Work out the finished part from the listing and answer in its coordinate system (mm). Face numbers are marked on the shaded views. A direction names the side the tool comes from. Round coordinates to 2 decimals unless told otherwise and drop trailing zeros. Order: outer loops, then holes, each group sorted by start corner. A loop starts at its lowest first (then second) coordinate and runs counter-clockwise, first axis right, second up. Notation, with made-up numbers: M -23.75,53.5 L 5.25,53.5 A17 cw 5.25,75.5 Z; hole C 55.25,-10.75 d10. An arc over 180 degrees is marked long. Return JSON: item names as keys, results as strings.
from build123d import *

# Parameters (mm, degrees)
ESQUISSE2_W                                    = 72
ESQUISSE2_H                                    = 14
BOSS_EXTRU_1_DEPTH                             = 41
ESQUISSE12_W                                   = 9
ESQUISSE12_H                                   = 20
BOSS_EXTRU_6_DEPTH                             = 14
FRAISAGE_POUR_VIS_T_TE_FRAIS_E_M41_D           = 4.3
FRAISAGE_POUR_VIS_T_TE_FRAIS_E_M41_CSINK_D     = 9.4
FRAISAGE_POUR_VIS_T_TE_FRAIS_E_M41_CSINK_ANGLE = 90
ENL_V_MAT_EXTRU_3_REACH                        = 95.798
ESQUISSE6_W                                    = 20
ESQUISSE6_H                                    = 10
ESQUISSE5_W                                    = 5.5
ESQUISSE5_H                                    = 50
ENL_V_MAT_EXTRU_2_DEPTH                        = 7
CHANFREIN1_SIZE                                = 2
ESQUISSE16_W                                   = 20
ESQUISSE16_H                                   = 7
BOSS_EXTRU_7_DEPTH                             = 10
ENL_V_START                                    = -14
ENL_V_MAT_EXTRU_4_DEPTH                        = 14
ENL_V_MAT_EXTRU_5_DEPTH                        = 7.5
CHANFREIN2_SIZE                                = 2
CONG_3_R                                       = 3


with BuildPart() as part:
    # Esquisse2 → Boss.-Extru.1 (new, symmetric)
    with BuildSketch(Plane.XY):
        Rectangle(ESQUISSE2_W, ESQUISSE2_H)
    extrude(amount=BOSS_EXTRU_1_DEPTH, both=True)

    # Esquisse12 → Boss.-Extru.6 (add)
    with BuildSketch(Plane(origin=(0, 7, 0), x_dir=(1, 0, 0), z_dir=(0, 1, 0))):
        with Locations((40.5, 0)):
            Rectangle(ESQUISSE12_W, ESQUISSE12_H)
    extrude(amount=-BOSS_EXTRU_6_DEPTH)

    # Fraisage pour vis à tête fraisée M41 (through all)
    with Locations(Plane(origin=(0, 7, 0), x_dir=(1, 0, 0), z_dir=(0, 1, 0))):
        with Locations((32.5, 0), (7.5, 0)):
            CounterSinkHole(FRAISAGE_POUR_VIS_T_TE_FRAIS_E_M41_D / 2, FRAISAGE_POUR_VIS_T_TE_FRAIS_E_M41_CSINK_D / 2, counter_sink_angle=FRAISAGE_POUR_VIS_T_TE_FRAIS_E_M41_CSINK_ANGLE)

    # Esquisse6 → Enlèv. mat.-Extru.3 (cut, up to next)
    with BuildSketch(Plane.XY.offset(41), mode=Mode.PRIVATE) as enl_v_mat_extru_3_sk1:
        with Locations((-18, -2)):
            Rectangle(ESQUISSE6_W, ESQUISSE6_H)
    enl_v_mat_extru_3_tool1 = extrude(enl_v_mat_extru_3_sk1.sketch, amount=-ENL_V_MAT_EXTRU_3_REACH, mode=Mode.PRIVATE) & part.part
    add(enl_v_mat_extru_3_tool1.solids().sort_by_distance((-18, -2, 41))[0], mode=Mode.SUBTRACT)

    # Esquisse5 → Enlèv. mat.-Extru.2 (cut)
    with BuildSketch(Plane(origin=(0, -7, 0), x_dir=(1, 0, 0), z_dir=(0, 1, 0))):
        with Locations((-33.25, 0)):
            Rectangle(ESQUISSE5_W, ESQUISSE5_H)
    extrude(amount=ENL_V_MAT_EXTRU_2_DEPTH, mode=Mode.SUBTRACT)

    # Chanfrein1
    chanfrein1_edges = [part.edges().sort_by_distance(p)[0] for p in [
        (0, 7, -41),
        (0, 7, 41),
    ]]
    chamfer(chanfrein1_edges, length=CHANFREIN1_SIZE)

    # Esquisse16 → Boss.-Extru.7 (add)
    with BuildSketch(Plane.XZ.offset(-3)):
        with Locations((-18, -37.5)):
            Rectangle(ESQUISSE16_W, ESQUISSE16_H)
    boss_extru_7 = extrude(amount=BOSS_EXTRU_7_DEPTH)

    # Symétrie1: Boss.-Extru.7 across plane
    add(boss_extru_7.mirror(Plane.XY))

    # Esquisse17 → Enlèv. mat.-Extru.4 (cut)
    with BuildSketch(Plane(origin=(0, 7, 0), x_dir=(1, 0, 0), z_dir=(0, 1, 0)).offset(ENL_V_START)):
        Polygon((13.342024655, -41), (21.739180223, -33.8), (7.912562911, -33.8), (-0.484592656, -41), align=None)
    extrude(amount=ENL_V_MAT_EXTRU_4_DEPTH, mode=Mode.SUBTRACT)

    # Esquisse18 → Enlèv. mat.-Extru.5 (cut)
    with BuildSketch(Plane(origin=(0, 7, 0), x_dir=(1, 0, 0), z_dir=(0, 1, 0))):
        Polygon((7.912562911, -33.8), (36, -10), (36, -21.716038419), (21.739180223, -33.8), align=None)
    extrude(amount=-ENL_V_MAT_EXTRU_5_DEPTH, mode=Mode.SUBTRACT)

    # Chanfrein2
    chanfrein2_edges = [part.edges().sort_by_distance(p)[0] for p in [
        (14.825871567, -0.5, 33.8),
        (36, -0.5, 15.858019209),
    ]]
    chamfer(chanfrein2_edges, length=CHANFREIN2_SIZE)

    # Congé3
    cong_3_edges = [part.edges().sort_by_distance(p)[0] for p in [
        (45, 0, 10),
        (45, 0, -10),
    ]]
    fillet(cong_3_edges, radius=CONG_3_R)


solid = part.part
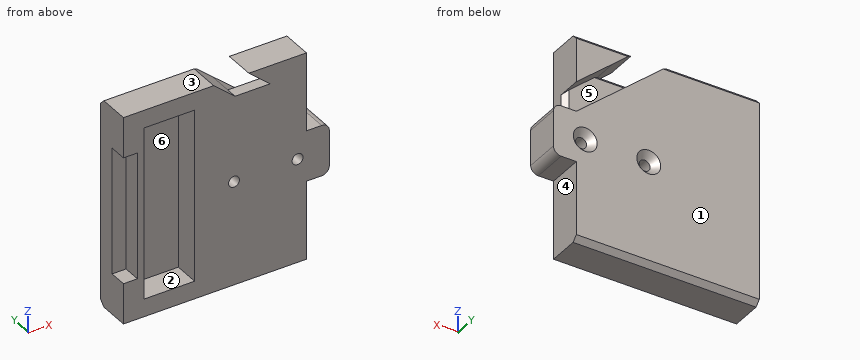
Item 1: Each of these flat-tipped pins is pushed along its axis until it touches: pin 1 (6 mm diameter, centred on x = 4, y = 1.5, fed in from +Z); pin 2 (5 mm diameter, centred on x = 39.5, y = -2, fed in from -Z); pin 3 (1.8 mm diameter, centred on x = 40, y = -0.5, fed in from +Z). Where does it stop, or does it pass through?
Output:
{"pin 1": "stops at z = 39.73", "pin 2": "stops at z = -10", "pin 3": "stops at z = 10"}
Item 2: Find section D-D (x = 32.5). Determine the outline of the cut face in (y, z), plus the area to 3 significant figures.
Output:
{"outline": "M -7,-41 L 5,-41 L 7,-39 L 7,-4.7 L 4.45,-2.15 L -7,-2.15 Z; M -7,2.15 L 4.45,2.15 L 7,4.7 L 7,12.97 L -0.5,12.97 L -0.5,24.68 L 7,24.68 L 7,39 L 5,41 L -7,41 Z", "area": "989 mm^2"}
Item 3: The mould has two halves that part along Z. Classify the marked faces 1, 2 and 3: pulls with the +Z half, pulls with the -Z half, needs draft (parallel to the pull), parting line crosses it, or undercut.
Output:
{"face 1": "needs draft", "face 2": "undercut", "face 3": "pulls with the +Z half"}
Item 4: Which of the six approach directions +Z, -Z, +X, -X, +Y, -Y give full straight-line access (tool end or side, diameter ignored) to the marked faces 4, 5 and 6?
Output:
{"face 4": "-Z, +X, +Y, -Y", "face 5": "+Y", "face 6": "-Y"}
Item 5: Find section A-A (y = 1.5). Determine the outline of the cut face in (x, z).
Output:
{"outline": "M -36,-41 L 36,-41 L 36,-10 L 42,-10 A3 ccw 45,-7 L 45,7 A3 ccw 42,10 L 36,10 L 7.91,33.8 L -0.48,41 L -36,41 Z; M 13.34,41 L 21.74,33.8 L 36,21.72 L 36,41 Z; hole M -28,-34 L -8,-34 L -8,34 L -28,34 Z; hole C 7.5,0 d4.3; hole C 32.5,0 d4.3"}
Item 6: Find section B-B (z = 0). Determine the outline of the cut face in (x, y).
Output:
{"outline": "M -36,0 L -30.5,0 L -30.5,-7 L -28,-7 L -28,3 L -8,3 L -8,-7 L 5.35,-7 L 5.35,4.45 L 2.8,7 L -36,7 Z; M 9.65,-7 L 30.35,-7 L 30.35,4.45 L 27.8,7 L 12.2,7 L 9.65,4.45 Z; M 34.65,-7 L 45,-7 L 45,7 L 37.2,7 L 34.65,4.45 Z"}
Item 7: Find section C-C (z = -19.5). Determine the outline of the cut face in (x, y), plus the area to 4 significant figures.
Output:
{"outline": "M -36,0 L -30.5,0 L -30.5,-7 L -28,-7 L -28,3 L -8,3 L -8,-7 L 36,-7 L 36,7 L -36,7 Z", "area": "769.5 mm^2"}
Item 8: Consider line 1 along Z through (x, y) = (32.5, 0.25); line 2 along Z through (x, y) = (32.5, -0.75); line 3 along Z through (x, y) = (-17, -2). Determine where each line is inside the solid, lowest interval first. Write a range as [from, to].
Output:
{"line 1": "z = [-41, -2.15], [2.15, 12.97], [24.68, 41]", "line 2": "z = [-41, -2.15], [2.15, 41]", "line 3": "z = [-41, -34], [34, 41]"}
